from build123d import *

# Parameters (mm, degrees)
F0_R            = 30
F0_R_2          = 26
F1_DEPTH        = 12
F2_W            = 8.4
F2_H            = 2.4
F3_DEPTH        = 11
F3_COPIES_COUNT = 15
F4_R            = 4.19999


# Not quite as in the source:
# - a fillet or chamfer is up to 0.001 mm smaller than in the source, because OpenCascade refuses the exact size
# - a pattern or mirror of a feature is missing from the dataset's text; its kind, count and spacing are read off the source's solid


with BuildPart() as f1:
    # F0 (on Top) → F1 (new body)
    with BuildSketch(Plane.XY):
        Circle(F0_R)
        Circle(F0_R_2, mode=Mode.SUBTRACT)
    extrude(amount=F1_DEPTH)

    # F2 (on face) → F3 (cut)
    with BuildSketch(Plane.XY.offset(12)):
        with Locations((0, 27.8)):
            Rectangle(F2_W, F2_H)
    f3 = extrude(amount=-F3_DEPTH, mode=Mode.SUBTRACT)

    # F3_copies: F3 ×15 about axis
    f3_copies_axis = Axis((0, 0, 0), (0, 0, 1))
    for i in range(1, F3_COPIES_COUNT):
        add(f3.rotate(f3_copies_axis, i * 360 / F3_COPIES_COUNT), mode=Mode.SUBTRACT)

    # F4 (radius 4.2 in the source; OpenCascade refuses exactly that, so slightly less here)
    f4_edges = [f1.edges().sort_by_distance(p)[0] for p in [
        (-4.2, 27.8, 1),
        (4.2, 27.8, 1),
        (-12.942559, -24.959371, 1),
        (-19.738301, -20.021974, 1),
        (-1.671725, -28.065732, 1),
        (-9.888165, -26.319274, 1),
        (-21.975506, -17.537307, 1),
        (-26.175506, -10.262693, 1),
        (-27.208689, -7.082883, 1),
        (-28.086728, 1.271101, 1),
        (9.888165, -26.319274, 1),
        (1.671725, -28.065732, 1),
        (19.738301, -20.021974, 1),
        (12.942559, -24.959371, 1),
        (26.175506, -10.262693, 1),
        (21.975506, -17.537307, 1),
        (28.086728, 1.271101, 1),
        (27.208689, -7.082883, 1),
        (-27.737243, 4.596235, 1),
        (-25.1415, 12.58511, 1),
        (-23.469775, 15.480623, 1),
        (-17.849078, 21.723039, 1),
        (-15.14417, 23.68827, 1),
        (-7.470388, 27.104858, 1),
        (25.1415, 12.58511, 1),
        (27.737243, 4.596235, 1),
        (15.14417, 23.68827, 1),
        (7.470388, 27.104858, 1),
        (17.849078, 21.723039, 1),
        (23.469775, 15.480623, 1),
    ]]
    fillet(f4_edges, radius=F4_R)


solid = f1.part
Verification items for the finished model (mm, model axes). Round coordinates to 2 decimals unless told otherwise and drop trailing zeros. Order: outer loops, then holes, each group sorted by start corner. A loop starts at its lowest first (then second) coordinate and runs counter-clockwise, first axis right, second up. Notation, with made-up numbers: (33, 59.25) -> (70, 59.25) arc R14 ccw to (70, 85.25) -> close; hole circle Ø10 at (-24, 76). An arc over 180 degrees is marked (long way). Put each result on its own line as item: value.
1) Material ranges on line 1 (Y direction, x = 0, z = 5); line 2 (X direction, y = 16, z = 10.75); line 3 (Y direction, x = 11.5, z = 9.75), recorded low to high.
Final values:
line 1: y = -30 to -26, 26 to 26.6, 29 to 30
line 2: x = -25.38 to -24.05, -21.39 to -20.49, 20.49 to 21.39, 24.05 to 25.38
line 3: y = -27.71 to -23.32, 23.32 to 24, 26.62 to 27.71
2) Depth check by flat-ended pin: pin 1 (6 mm diameter, centred on x = -19, z = 8, fed in from -Y); pin 2 (4 mm diameter, centred on y = 18.5, z = 7, fed in from -X); pin 3 (1.1 mm diameter, centred on x = 16.5, y = -22, fed in from +Z). Enter the tip coordinate at first touch or a pass-through.
Final values:
pin 1: stops at y = -25.38
pin 2: stops at x = -25.05
pin 3: stops at z = 1.11
3) Section check B-B (z = 11.25). Give the number of separate pieces and of enclosed holes in the cut face, then the cut area to 3 significant figures.
Final values:
separate pieces: 1
enclosed holes: 16
area: 401 mm^2
4) Section check A-A (y = 2.5). Record the cut outline in (x, z).
Final values:
outline: (-29.9, 0) -> (-25.88, 0) -> (-25.88, 12) -> (-29.9, 12) -> close; (25.88, 0) -> (29.9, 0) -> (29.9, 12) -> (25.88, 12) -> close
5) Mould release check, pull along X, two halves, no side actions. Record for faces 1 (the flat face through (6.087, -28.354, 6.577)), 2 (the cylindrical face through (-8.72, -26.585, 2.263)): +X half, -X half, draft (parallel to the pull), parting line (faces both ways), or undercut.
Final values:
face 1: undercut
face 2: undercut
